Part model, mm, in its own coordinate system. Face numbers are marked on the shaded views. A direction names the side the tool comes from. Give positions to 0.01 mm unless a question says otherwise; leave off trailing zeros. Order: outer loops, then holes, each group sorted by start corner. A loop starts at its lowest first (then second) coordinate and runs counter-clockwise, first axis right, second up. Notation, with made-up numbers: (17, -17) -> (67, -17) arc R26 cw to (67, 13) -> close; hole circle Ø3 at (0.25, 70.5). An arc over 180 degrees is marked (long way). Write item = value, one per line. Start each with the question number.
(1) Which spindle directions (+Z, -Z, +X, -X, +Y, -Y) get a long thin tool onto all of the face, cutting with end or side? Do the marked faces 1 and 2. Say none if no direction does.
(2) Saw through at C-C, the plane x = 0. List the corners of the cut face in (y, z) (3 decimals).
(3) Saw through at A-A, the plane y = -2.25. List the corners of the cut face in (x, z) (3 decimals).
(4) Saw through at B-B, the plane z = -15.24. List the corners of the cut face in (x, y) (3 decimals), then the cut area to 3 significant figures.
(5) Flat gauge pins, fed straight in: pin 1 (3.5 mm diameter, centred on x = 0, z = -15.24, fed in from +Y); pin 2 (19 mm diameter, centred on x = -7, z = -29.5, fed in from -Y). Where does each tip first touch, or does it go through?
(6) Probe line 1 along Z through (x, y) = (0, -0.85) (3 decimals); line 2 along Z through (x, y) = (0, -6) (3 decimals); line 3 along Y through (x, z) = (-10, -51.5). List the from-to ranges inside material, lowest first. Write a range as from..to.
(7) Saw through at D-D, the plane x = 4.5. List the corners of the cut face in (y, z) (3 decimals), then the cut area to 3 significant figures.
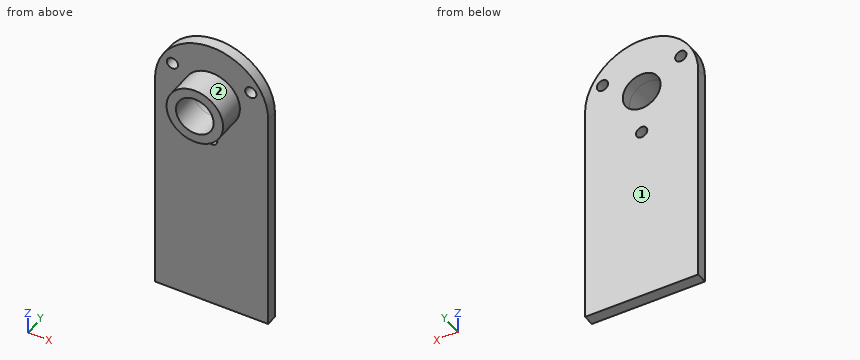
Autodesk Inventor part; units mm, degrees
ref_plane "YZ Plane" through (0, 0, 0) normal (1, 0, 0) x (0, 1, 0)
ref_plane "XZ Plane" through (0, 0, 0) normal (0, 1, 0) x (-1, 0, 0)
ref_plane "XY Plane" through (0, 0, 0) normal (0, 0, 1) x (1, 0, 0)
sketch "Sketch1" plane through (0, 0, 0) normal (0, 1, 0) x (-1, 0, 0)
  circle A0 centre (0, 0) radius 15.24 construction
  circle A1 centre (0, -15.24) radius 1.905
  circle A2 centre (13.1982, 7.62) radius 1.905
  circle A3 centre (-13.1982, 7.62) radius 1.905
  arc A4 (19.05, 0) -> (-19.05, 0) centre (0, 0) ccw
  line L0 (19.05, 0) -> (19.05, -76.2)
  line L1 (19.05, -76.2) -> (-19.05, -76.2)
  line L2 (-19.05, -76.2) -> (-19.05, 0)
  circle A5 centre (0, 0) radius 6.35
  point P0 (0, -19.05)
  point P1 (0, 19.05)
  dimension "boltHoleDiameter" = 30.48
  dimension "d1" = 3.81
  dimension "d4" = 360
  dimension "exteriorOfBolts" = 38.1
  dimension "majorLength" = 76.2
  dimension "d12" = 12.7
extrude "Extrusion2" add sketch "Sketch1" against normal blind 3.81
sketch "Sketch2" plane through (0, -3.81, 0) normal (0, -1, 0) x (1, 0, 0)
  circle A0 centre (0, 0) radius 6.35
  circle A1 centre (0, 0) radius 9.525
  dimension "d15" = 19.05
extrude "Extrusion3" add sketch "Sketch2" along normal blind 9.525
properties part number "Focuser Base"
Results list:
q1.face_1 = +Z, -Z, +X, -X, +Y
q1.face_2 = -Y
q2.outline = (-13.335, -9.525) -> (-3.81, -9.525) -> (-3.81, -13.335) -> (0, -13.335) -> (0, -6.35) -> (-13.335, -6.35) -> close; (-13.335, 6.35) -> (0, 6.35) -> (0, 19.05) -> (-3.81, 19.05) -> (-3.81, 9.525) -> (-13.335, 9.525) -> close; (-3.81, -76.2) -> (0, -76.2) -> (0, -17.145) -> (-3.81, -17.145) -> close
q3.outline = (-19.05, -76.2) -> (19.05, -76.2) -> (19.05, 0) arc R19.05 ccw to (-19.05, 0) -> close; hole circle Ø3.81 at (-13.198, 7.62); hole circle Ø12.7 at (0, 0); hole circle Ø3.81 at (0, -15.24); hole circle Ø3.81 at (13.198, 7.62)
q4.outline = (-19.05, -3.81) -> (-1.905, -3.81) -> (-1.905, 0) -> (-19.05, 0) -> close; (1.905, -3.81) -> (19.05, -3.81) -> (19.05, 0) -> (1.905, 0) -> close
q4.area = 131 mm^2
q5.pin_1 = through
q5.pin_2 = -3.81
q6.line_1 = -76.2..-17.145, -13.335..-6.35, 6.35..19.05
q6.line_2 = -9.525..-6.35, 6.35..9.525
q6.line_3 = -3.81..0
q7.outline = (-13.335, -8.395) -> (-3.81, -8.395) -> (-3.81, -76.2) -> (0, -76.2) -> (0, -4.48) -> (-13.335, -4.48) -> close; (-13.335, 4.48) -> (0, 4.48) -> (0, 18.511) -> (-3.81, 18.511) -> (-3.81, 8.395) -> (-13.335, 8.395) -> close
q7.area = 401 mm^2
